Study the drawing (mm; zero at the part's minimum x, y, z) and answer. A direction names the side the tool comes from. Round coordinates to 2 decimals unless told otherwise and drop trailing zeros. Write each loop counter-clockwise with the first axis right and the second up, starting at its lowest first coordinate (ties: lowest second). Pieces come first, ordered by that corner, then holes.
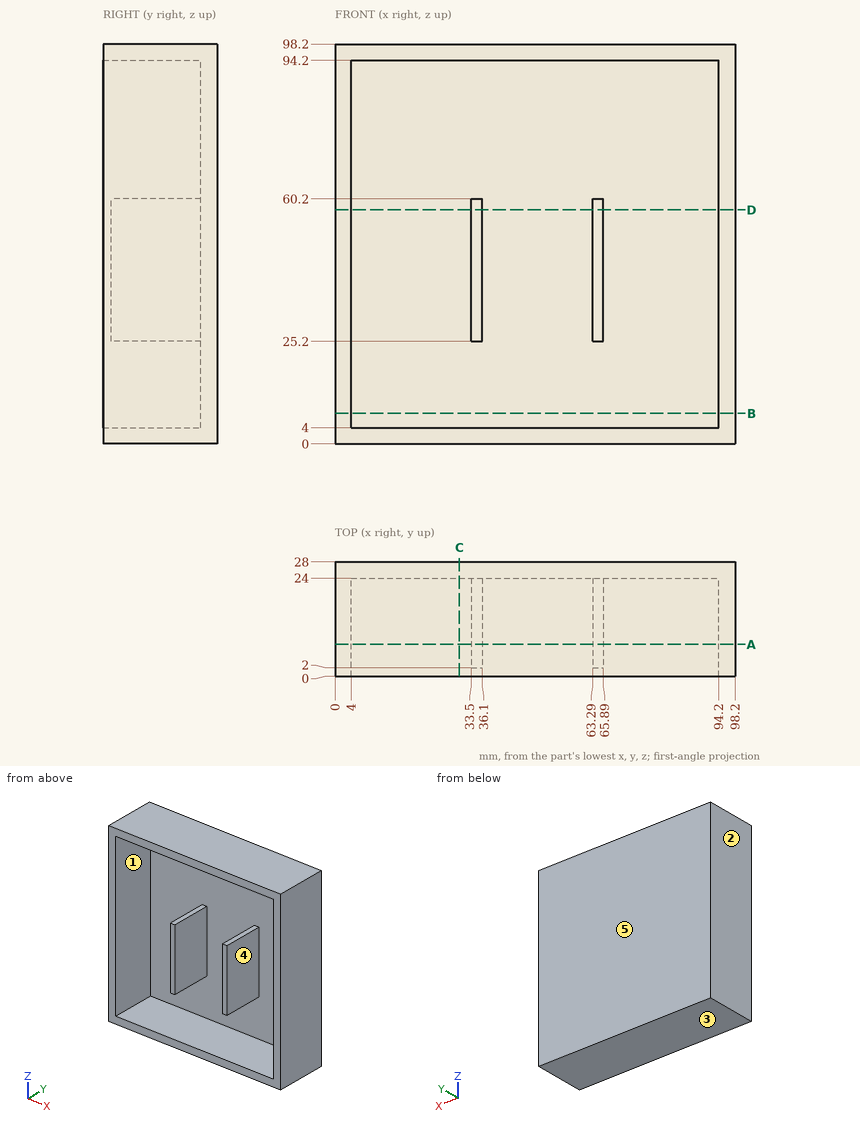
Q1. Find section B-B (z = 7.5). Determine the outline of the cut face in (x, y), plus the area to 3 significant figures.
Q2. Find the intervals of material crossed by L1, parallel to X at y = 20, z = 41; L2, parallel to Z at x = 34, y = 4.5; L3, parallel to Z at x = 25.5, y = 15.75, in increasing order.
Q3. Given pin 1 (4 mm diameter, centred on x = 44, z = 29.5, fed in from -Y); pin 2 (2 mm diameter, centred on x = 34.5, z = 39.5, fed in from -Y), each flat-ended and moving along its own axis, determine where each tip first touches the part or whether it passes through.
Q4. The mould has two halves that part along Z. Classify the marked faces 3, 4 and 5: +Z half, -Z half, draft (parallel to the pull), parting line (faces both ways), or undercut.
Q5. Find section C-C (x = 30.5). Determine the outline of the cut face in (y, z), plus the area to 3 significant figures.
Q6. Find section A-A (y = 7.75). Determine the outline of the cut face in (x, z).
Q7. Find section D-D (z = 57.5). Determine the outline of the cut face in (x, y), plus the area to 3 significant figures.
Q8. A tool of negligible diameter and unlimited length cuts with its end or side. For the marked faces 1 and 2, from which of +Z, -Z, +X, -X, +Y, -Y can it reach the whole face along a straight path? Write none if from no direction.
Report:
1. outline: (0, 0) - (4, 0) - (4, 24) - (94.2, 24) - (94.2, 0) - (98.2, 0) - (98.2, 28) - (0, 28) - close
1. area: 585 mm2
2. L1: x = 0 to 4, 33.5 to 36.1, 63.29 to 65.89, 94.2 to 98.2
2. L2: z = 0 to 4, 25.2 to 60.2, 94.2 to 98.2
2. L3: z = 0 to 4, 94.2 to 98.2
3. pin 1: stops at y = 24
3. pin 2: stops at y = 2
4. face 3: -Z half
4. face 4: undercut
4. face 5: draft
5. outline: (0, 0) - (28, 0) - (28, 98.2) - (0, 98.2) - (0, 94.2) - (24, 94.2) - (24, 4) - (0, 4) - close
5. area: 585 mm2
6. outline: (0, 0) - (98.2, 0) - (98.2, 98.2) - (0, 98.2) - close; (33.5, 25.2) - (36.1, 25.2) - (36.1, 60.2) - (33.5, 60.2) - close; (63.29, 25.2) - (65.89, 25.2) - (65.89, 60.2) - (63.29, 60.2) - close; hole (4, 4) - (94.2, 4) - (94.2, 94.2) - (4, 94.2) - close
7. outline: (0, 0) - (4, 0) - (4, 24) - (33.5, 24) - (33.5, 2) - (36.1, 2) - (36.1, 24) - (63.29, 24) - (63.29, 2) - (65.89, 2) - (65.89, 24) - (94.2, 24) - (94.2, 0) - (98.2, 0) - (98.2, 28) - (0, 28) - close
7. area: 699 mm2
8. face 1: -Y
8. face 2: +Z, -Z, -X, +Y, -Y
